Autodesk Inventor part; units mm, degrees
ref_plane "YZ Plane" through (0, 0, 0) normal (1, 0, 0) x (0, 1, 0)
ref_plane "XZ Plane" through (0, 0, 0) normal (0, 1, 0) x (-1, 0, 0)
ref_plane "XY Plane" through (0, 0, 0) normal (0, 0, 1) x (1, 0, 0)
sketch "Sketch1" plane through (0, 0, 0) normal (0, 0, 1) x (1, 0, 0)
  line L0 (-12.1708, 16.0073) -> (13.2292, 16.0073)
  line L1 (13.2292, 16.0073) -> (13.2292, -34.7927)
  line L2 (13.2292, -34.7927) -> (-12.1708, -34.7927)
  line L3 (-12.1708, -34.7927) -> (-12.1708, 16.0073)
  line L4 (11.9592, 14.7373) -> (-10.9008, 14.7373)
  line L5 (-10.9008, 14.7373) -> (-10.9008, -33.5227)
  line L6 (-10.9008, -33.5227) -> (11.9592, -33.5227)
  line L7 (11.9592, -33.5227) -> (11.9592, 14.7373)
  point P0 (0, 0)
  dimension "d0" = 25.4
  dimension "d1" = 50.8
  dimension "d2" = 1.27
extrude "Extrusion1" add sketch "Sketch1" along normal blind 635
sketch "Sketch2" plane through (-12.1708, 16.0073, 0) normal (0, 1, 0) x (1, 0, 0)
  circle A0 centre (12.7, -12.7) radius 1.7272
  line L0 (25.4, 0) -> (0, 0)
  line L1 (0, 0) -> (0, -635)
  point P0 (12.1708, 0)
  dimension "d5" = 3.4544
  dimension "d6" = 12.7
  dimension "d7" = 12.7
extrude "Extrusion2" cut sketch "Sketch2" against normal through all
pattern_linear "Rectangular Pattern1" count 64 spacing 25.4 along (0, 0, 1) of "Extrusion2"
equation "\"d3\" = d13"
equation "\"d10\" = d14"
equation "\"d13\" = 635"
equation "\"d14\" = d13"
properties part number "VersaFrame (PerimeterPieceA)"
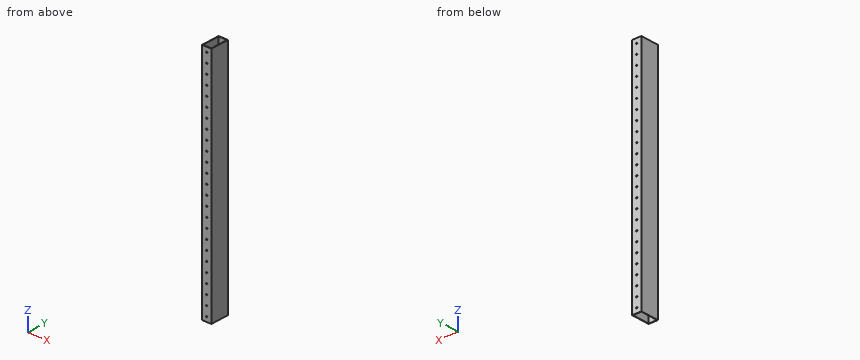
For this review, take the finished solid that the model builds, in its own axes (mm). Coordinates: 2 decimals unless noted, no trailing zeros. Write each loop counter-clockwise with the first axis right and the second up, starting at its lowest first coordinate (ties: lowest second). Pieces come first, ordered by that corner, then holes. Notation, with made-up numbers: (55.25, -24) - (113.25, -24) arc R33 cw to (113.25, 14) - close; hole circle Ø7 at (15, 89.25). An arc over 180 degrees is marked (long way). Answer in a Markdown table with one row per item. Add a question column.
Q1. For probe 1 along Y at (x, z) = (-8, 263); probe 2 along X at (y, z) = (10, 376); probe 3 along X at (y, z) = (15.15, 190.5), list the stretches that pass through material, from the lowest coordinate up.
Q2. We need section B-B, the plane x = 6.75. State the section outline as (y, z) points, and give its area (3 significant figures).
Q3. We need section A-A, the plane y = -14.5. State the section outline as (x, z) points.
Q4. We need section C-C, the plane z = 177.5. State the section outline as (x, y) points, and give its area (3 significant figures).
Q5. For P1, Ø5.5, axis at x = 0.53, z = 393.7, coming from the +Y side, flat-tipped, find the tip position at first contact; note if it passes through.
Answer list:
| question | item | result |
|---|---|---|
| 1 | probe 1 | y = -34.79 to -33.52, 14.74 to 16.01 |
| 1 | probe 2 | x = -12.17 to -10.9, 11.96 to 13.23 |
| 1 | probe 3 | x = -12.17 to -1.2, 2.26 to 13.23 |
| 2 | outline | (-34.79, 0) - (-33.52, 0) - (-33.52, 635) - (-34.79, 635) - close; (14.74, 0) - (16.01, 0) - (16.01, 635) - (14.74, 635) - close |
| 2 | area | 1,610 mm2 |
| 3 | outline | (-12.17, 0) - (-10.9, 0) - (-10.9, 635) - (-12.17, 635) - close; (11.96, 0) - (13.23, 0) - (13.23, 635) - (11.96, 635) - close |
| 4 | outline | (-12.17, -34.79) - (13.23, -34.79) - (13.23, 16.01) - (-12.17, 16.01) - close; hole (-10.9, -33.52) - (11.96, -33.52) - (11.96, 14.74) - (-10.9, 14.74) - close |
| 4 | area | 187 mm2 |
| 5 | P1 | stops at y = 16.01 |
